Can you work these out from the model? Positions are in its coordinate system, mm. Give positions to 0.01 mm unless a question says otherwise; leave off trailing zeros. Order: outer loops, then holes, each group sorted by start corner. A loop starts at its lowest first (then second) coordinate and runs counter-clockwise, first axis right, second up. Notation, with made-up numbers: (7, 88.25) - (19, 88.25) arc R17 cw to (19, 115.25) - close; hole circle Ø6 at (-8, 52.25). An arc over 180 degrees is marked (long way). One line per question, with ' | ' between items.
```python
from build123d import *

# Parameters (mm, degrees)
F0_W     = 390
F0_H     = 80
F0_R     = 4.75
F1_DEPTH = 30
F2_W     = 390
F2_H     = 80
F3_DEPTH = 25


with BuildPart() as f1:
    # F0 (on Top) → F1 (new body)
    with BuildSketch(Plane.XY):
        with Locations((175, 24.758239)):
            Rectangle(F0_W, F0_H)
        with BuildLine():
            ThreePointArc((-4.1265, 2.352552), (-2.397378, 4.100619), (-0.02588, 4.749929))
            ThreePointArc((-0.02588, 4.749929), (2.352552, 4.1265), (4.100619, 2.397378))
            ThreePointArc((4.100619, 2.397378), (4.584781, 1.241885), (4.75, 0))
            ThreePointArc((4.75, 0), (4.59148, -1.216887), (4.1265, -2.352552))
            ThreePointArc((4.1265, -2.352552), (2.397378, -4.100619), (0.02588, -4.749929))
            ThreePointArc((0.02588, -4.749929), (-2.352552, -4.1265), (-4.100619, -2.397378))
            ThreePointArc((-4.100619, -2.397378), (-4.749929, -0.02588), (-4.1265, 2.352552))
        make_face(mode=Mode.SUBTRACT)
        with Locations((25, 0)):
            Circle(F0_R, mode=Mode.SUBTRACT)
        with Locations((50, 0)):
            Circle(F0_R, mode=Mode.SUBTRACT)
        with Locations((75, 0)):
            Circle(F0_R, mode=Mode.SUBTRACT)
        with Locations((100, 0)):
            Circle(F0_R, mode=Mode.SUBTRACT)
        with Locations((125, 0)):
            Circle(F0_R, mode=Mode.SUBTRACT)
        with Locations((150, 0)):
            Circle(F0_R, mode=Mode.SUBTRACT)
        with Locations((175, 0)):
            Circle(F0_R, mode=Mode.SUBTRACT)
        with Locations((200, 0)):
            Circle(F0_R, mode=Mode.SUBTRACT)
        with Locations((225, 0)):
            Circle(F0_R, mode=Mode.SUBTRACT)
        with Locations((250, 0)):
            Circle(F0_R, mode=Mode.SUBTRACT)
        with Locations((275, 0)):
            Circle(F0_R, mode=Mode.SUBTRACT)
        with Locations((300, 0)):
            Circle(F0_R, mode=Mode.SUBTRACT)
        with Locations((325, 0)):
            Circle(F0_R, mode=Mode.SUBTRACT)
        with Locations((350, 0)):
            Circle(F0_R, mode=Mode.SUBTRACT)
        with Locations((0, 25)):
            Circle(F0_R, mode=Mode.SUBTRACT)
        with Locations((25, 25)):
            Circle(F0_R, mode=Mode.SUBTRACT)
        with Locations((50, 25)):
            Circle(F0_R, mode=Mode.SUBTRACT)
        with Locations((75, 25)):
            Circle(F0_R, mode=Mode.SUBTRACT)
        with Locations((100, 25)):
            Circle(F0_R, mode=Mode.SUBTRACT)
        with Locations((125, 25)):
            Circle(F0_R, mode=Mode.SUBTRACT)
        with Locations((150, 25)):
            Circle(F0_R, mode=Mode.SUBTRACT)
        with Locations((0, 50)):
            Circle(F0_R, mode=Mode.SUBTRACT)
        with Locations((25, 50)):
            Circle(F0_R, mode=Mode.SUBTRACT)
        with Locations((50, 50)):
            Circle(F0_R, mode=Mode.SUBTRACT)
        with Locations((75, 50)):
            Circle(F0_R, mode=Mode.SUBTRACT)
        with Locations((100, 50)):
            Circle(F0_R, mode=Mode.SUBTRACT)
        with Locations((125, 50)):
            Circle(F0_R, mode=Mode.SUBTRACT)
        with Locations((150, 50)):
            Circle(F0_R, mode=Mode.SUBTRACT)
        with Locations((175, 25)):
            Circle(F0_R, mode=Mode.SUBTRACT)
        with Locations((200, 25)):
            Circle(F0_R, mode=Mode.SUBTRACT)
        with Locations((225, 25)):
            Circle(F0_R, mode=Mode.SUBTRACT)
        with Locations((250, 25)):
            Circle(F0_R, mode=Mode.SUBTRACT)
        with Locations((275, 25)):
            Circle(F0_R, mode=Mode.SUBTRACT)
        with Locations((300, 25)):
            Circle(F0_R, mode=Mode.SUBTRACT)
        with Locations((325, 25)):
            Circle(F0_R, mode=Mode.SUBTRACT)
        with Locations((350, 25)):
            Circle(F0_R, mode=Mode.SUBTRACT)
        with Locations((175, 50)):
            Circle(F0_R, mode=Mode.SUBTRACT)
        with Locations((200, 50)):
            Circle(F0_R, mode=Mode.SUBTRACT)
        with Locations((225, 50)):
            Circle(F0_R, mode=Mode.SUBTRACT)
        with Locations((250, 50)):
            Circle(F0_R, mode=Mode.SUBTRACT)
        with Locations((275, 50)):
            Circle(F0_R, mode=Mode.SUBTRACT)
        with Locations((300, 50)):
            Circle(F0_R, mode=Mode.SUBTRACT)
        with Locations((325, 50)):
            Circle(F0_R, mode=Mode.SUBTRACT)
        with Locations((350, 50)):
            Circle(F0_R, mode=Mode.SUBTRACT)
    extrude(amount=F1_DEPTH)

    # F2 (on face) → F3 (join)
    with BuildSketch(Plane(origin=(0, 0, 0), x_dir=(1, 0, 0), z_dir=(0, 0, -1))):
        with Locations((175, -24.758239)):
            Rectangle(F2_W, F2_H)
    extrude(amount=F3_DEPTH)


solid = f1.part
```
(1) Will these pins go through, and if not, where does the flat tip stop? pin 1 (3 mm diameter, centred on x = 77, y = 25, fed in from +Z); pin 2 (15 mm diameter, centred on x = 50, y = 25, fed in from +Z).
Answer below:
pin 1: z = 0 | pin 2: z = 30
(2) Imagine slicing it at B-B (z = 6). Count the separate pieces of the cut face and the enclosed holes in it, and give its area (3 significant figures).
Answer below:
separate pieces: 1 | enclosed holes: 45 | area: 28,000 mm^2
(3) If I drill on line 1 (Y direction, x = 250, z = 22); line 2 (Y direction, x = 29, z = 15); line 3 (Z direction, x = 151, y = 48), over which ranges is the centre line in solid material (lowest first)?
Answer below:
line 1: -15.24 to -4.75, 4.75 to 20.25, 29.75 to 45.25, 54.75 to 64.76 | line 2: -15.24 to -2.56, 2.56 to 22.44, 27.56 to 47.44, 52.56 to 64.76 | line 3: -25 to 0
(4) Imagine slicing it at A-A (x = 25). List the corners of the cut face in (y, z) for me, and give its area (4 significant figures).
Answer below:
outline: (-15.24, -25) - (64.76, -25) - (64.76, 30) - (54.75, 30) - (54.75, 0) - (45.25, 0) - (45.25, 30) - (29.75, 30) - (29.75, 0) - (20.25, 0) - (20.25, 30) - (4.75, 30) - (4.75, 0) - (-4.75, 0) - (-4.75, 30) - (-15.24, 30) - close | area: 3,545 mm^2
